Check sheet for the modelled part. Datum: model origin and axes. Units: mm. A direction names the side the tool comes from. Round coordinates to 2 decimals unless told otherwise and drop trailing zeros. Loops run counter-clockwise (first coordinate to the right, second up) from the corner with the lowest first, then second, coordinate; pieces in that order, holes last. Notation, with made-up numbers: (11, -0.5) - (18, -0.5) arc R25 ccw to (18, 35.5) - close; hole circle Ø9 at (-18.5, -29). An arc over 180 degrees is marked (long way). Put each result on its own line as item: value. Start each with the question number.
Item 1: Section check A-A, the plane y = -4.5. Record the cut outline in (x, z), and give its area (3 significant figures).
Item 2: Section check C-C, the plane z = 4.5. Record the cut outline in (x, y).
Item 3: Gauge pin test, flat ends, axial feed: pin 1 Ø1.5 at (x, y) = (1, -5.5) entering from +Z; pin 2 Ø0.6 at (y, z) = (-1, 0) entering from -X; pin 3 Ø3 at (y, z) = (-4, -4.5) entering from +X; pin 4 Ø1.5 at (x, y) = (-2, -1) entering from -Z. Record the tip position at first contact, or that the pin passes through.
Item 4: Tool access check on faces 4 (the flat face through (0, -3, -0.394)), 5 (the flat face through (0, 0.254, 0)). Record the directions out of +Z, -Z, +X, -X, +Y, -Y that give a thin tool (end or side, any length) a straight path to the whole face; none if there is none.
Item 5: Draft check along Z on faces 1 (the flat face through (0, -3, 0.394)), 2 (the flat face through (0, -3, -5.093)), 3 (the flat face through (0, -3, 5.093)). Enter one of: pulls with the +Z half, pulls with the -Z half, needs draft (parallel to the pull), parting line crosses it, or undercut.
Item 6: Section check D-D, the plane y = -1.25. Record the cut outline in (x, z).
Item 7: Material ranges on line 1 along Z through (x, y) = (0, -6.25); line 2 along Y through (x, z) = (-1.75, 0.5); line 3 along X through (y, z) = (-5, -5), recorded low to high.
Item 8: Section check B-B, the plane x = 0. Record the cut outline in (y, z).
Autodesk Inventor part; units mm, degrees
ref_plane "to_base_XY" through (0, 0, 0) normal (0, 1, 0) x (1, 0, 0)
ref_plane "to_base_YZ" through (0, 0, 0) normal (1, 0, 0) x (0, 0, -1)
ref_plane "to_base_ZX" through (0, 0, 0) normal (0, 0, -1) x (0, 1, 0)
sketch "Sketch_2" plane through (0, 0, 0) normal (0, 1, 0) x (-1, 0, 0)
  line L0 (3.1877, -6.1184) -> (3.1877, 6.1184)
  arc A0 (3.1877, 6.1184) -> (3.0577, 6.2484) centre (3.0577, 6.1184) ccw
  line L1 (3.0577, 6.2484) -> (-3.0577, 6.2484)
  arc A1 (-3.0577, 6.2484) -> (-3.1877, 6.1184) centre (-3.0577, 6.1184) ccw
  line L2 (-3.1877, 6.1184) -> (-3.1877, -6.1184)
  arc A2 (-3.1877, -6.1184) -> (-3.0577, -6.2484) centre (-3.0577, -6.1184) ccw
  line L3 (-3.0577, -6.2484) -> (3.0577, -6.2484)
  arc A3 (3.0577, -6.2484) -> (3.1877, -6.1184) centre (3.0577, -6.1184) ccw
extrude "Extrusion1" add sketch "Sketch_2" along normal blind 0.254
sketch "Sketch_7" plane through (0, 0, -4.699) normal (0, 0, 1) x (1, 0, 0)
  line L0 (-0.9271, 0) -> (-0.9271, -1.8034)
  line L1 (-0.9271, -1.8034) -> (-0.5842, -1.8034)
  line L2 (-0.5842, -1.8034) -> (-0.5842, -6.0198)
  arc A0 (-0.5842, -6.0198) -> (0.5842, -6.0198) centre (0, -6.0198) ccw
  line L3 (0.5842, -6.0198) -> (0.5842, -1.8034)
  line L4 (0.5842, -1.8034) -> (0.9271, -1.8034)
  line L5 (0.9271, -1.8034) -> (0.9271, 0)
  line L6 (0.9271, 0) -> (-0.9271, 0)
extrude "Extrusion2" add sketch "Sketch_7" along normal mid plane 0.7874
pattern_linear "Rectangular Pattern1" count 3 spacing 4.699 along (0, 0, 1) of "Extrusion2"
ref_plane "to_base_XY" through (0, 0, 0) normal (0, 1, 0) x (1, 0, 0)
ref_plane "to_base_YZ" through (0, 0, 0) normal (1, 0, 0) x (0, 0, -1)
ref_plane "to_base_ZX" through (0, 0, 0) normal (0, 0, -1) x (0, 1, 0)
properties part number "M201503-terminals"
Check result:
1. outline: (-0.58, -5.09) - (0.58, -5.09) - (0.58, -4.31) - (-0.58, -4.31) - close; (-0.58, -0.39) - (0.58, -0.39) - (0.58, 0.39) - (-0.58, 0.39) - close; (-0.58, 4.31) - (0.58, 4.31) - (0.58, 5.09) - (-0.58, 5.09) - close
1. area: 2.76 mm²
2. outline: (-3.19, 0) - (-0.93, 0) - (-0.93, -1.8) - (-0.58, -1.8) - (-0.58, -6.02) arc R0.58 ccw to (0.58, -6.02) - (0.58, -1.8) - (0.93, -1.8) - (0.93, 0) - (3.19, 0) - (3.19, 0.25) - (-3.19, 0.25) - close
3. pin 1: z = 5.09
3. pin 2: x = -0.93
3. pin 3: x = 0.58
3. pin 4: through
4. face 4: +X, -X, -Y
4. face 5: +Z, -Z, +X, -X, +Y
5. face 1: undercut
5. face 2: pulls with the -Z half
5. face 3: pulls with the +Z half
6. outline: (-0.93, -5.09) - (0.93, -5.09) - (0.93, -4.31) - (-0.93, -4.31) - close; (-0.93, -0.39) - (0.93, -0.39) - (0.93, 0.39) - (-0.93, 0.39) - close; (-0.93, 4.31) - (0.93, 4.31) - (0.93, 5.09) - (-0.93, 5.09) - close
7. line 1: -5.09 to -4.31, -0.39 to 0.39, 4.31 to 5.09
7. line 2: 0 to 0.25
7. line 3: -0.58 to 0.58
8. outline: (-6.6, -5.09) - (0, -5.09) - (0, -6.25) - (0.25, -6.25) - (0.25, 6.25) - (0, 6.25) - (0, 5.09) - (-6.6, 5.09) - (-6.6, 4.31) - (0, 4.31) - (0, 0.39) - (-6.6, 0.39) - (-6.6, -0.39) - (0, -0.39) - (0, -4.31) - (-6.6, -4.31) - close
